Part print with two shaded views. Sizes in mm from the minimum x, y, z corner. Give positions to 0.01 mm unless a question says otherwise; leave off trailing zeros. Order: outer loops, then holes, each group sorted by start corner. A loop starts at its lowest first (then second) coordinate and runs counter-clockwise, first axis right, second up. Notation, with made-up numbers: M 39,44.5 L 98,44.5 A22 ccw 98,77.5 Z; hole C 11.5,81 d1. An arc over 180 degrees is marked long. Answer as CSV lines item,"result".
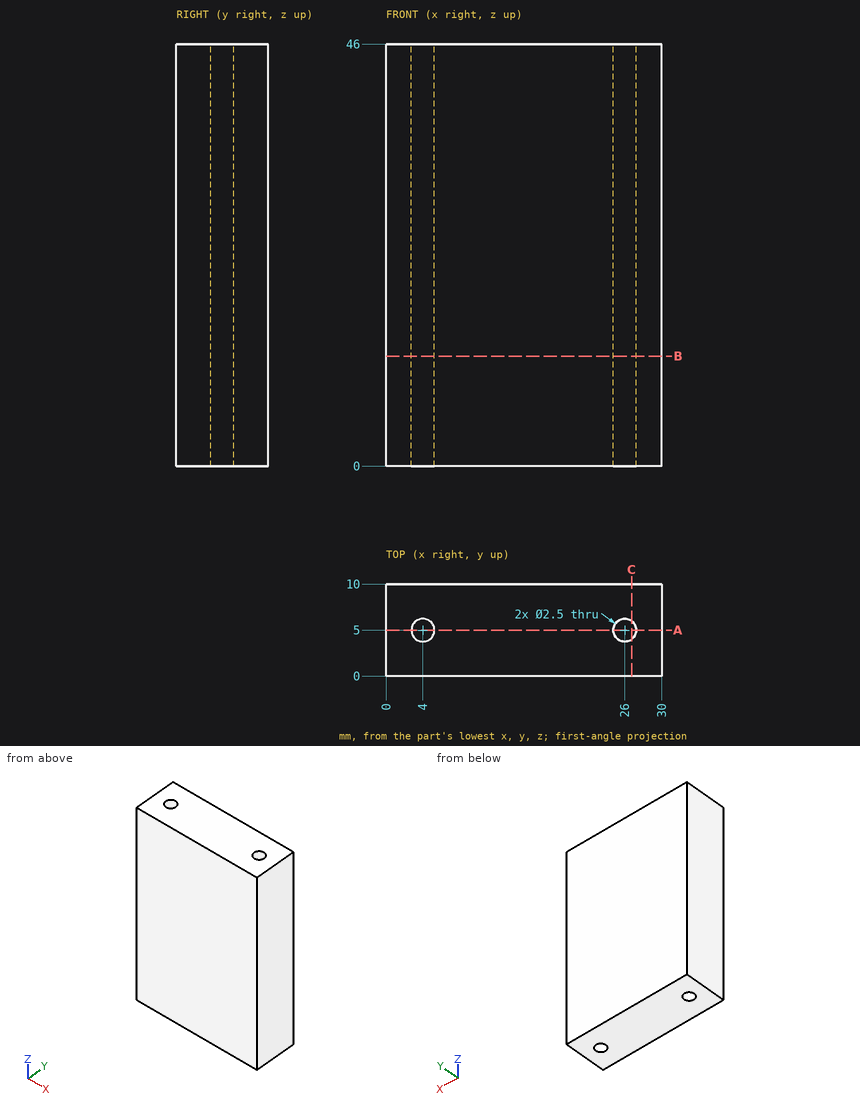
Item 1: Band-saw the part on C-C (x = 26.75). Give the cut face in (y, z), and give its area (3 significant figures).
Geometry says:
outline,"M 0,0 L 4,0 L 4,46 L 0,46 Z; M 6,0 L 10,0 L 10,46 L 6,46 Z"
area,"368 mm2"
Item 2: Drop a flat-ended pin along its axis: pin 1 (2 mm diameter, centred on x = 4, y = 5, fed in from -Z). Give the stop position or say it passes through.
Geometry says:
pin 1,"passes through"
Item 3: Band-saw the part on A-A (y = 5). Give the cut face in (x, z).
Geometry says:
outline,"M 0,0 L 2.75,0 L 2.75,46 L 0,46 Z; M 5.25,0 L 24.75,0 L 24.75,46 L 5.25,46 Z; M 27.25,0 L 30,0 L 30,46 L 27.25,46 Z"
Item 4: Band-saw the part on B-B (z = 12). Give the cut face in (x, y).
Geometry says:
outline,"M 0,0 L 30,0 L 30,10 L 0,10 Z; hole C 4,5 d2.5; hole C 26,5 d2.5"
Item 5: Probe line 1 along X through (y, z) = (5, 36); line 2 along Y through (x, z) = (26, 15); line 3 along X through (y, z) = (4, 40.5). List the from-to ranges inside material, lowest first. Write a range as from..to.
Geometry says:
line 1,"x = 0..2.75, 5.25..24.75, 27.25..30"
line 2,"y = 0..3.75, 6.25..10"
line 3,"x = 0..3.25, 4.75..25.25, 26.75..30"
